Source: CAD feature listing. Evaluate the final solid. Frame: model axes, mm. A direction names the side the tool comes from. Coordinates: 2 decimals unless noted, no trailing zeros. Write each loop counter-clockwise with the first axis right and the second up, starting at its lowest first coordinate (ties: lowest second). Pieces come first, ordered by that corner, then holes. Notation, with made-up numbers: (-28.5, 10) - (-8.5, 10) arc R25 cw to (-8.5, 39) - close; hole circle Ø8 at (68.5, 86.5). An arc over 180 degrees is marked (long way). One line per question, with ' | ' between items. Start each with the question number.
Q1. Line query: line 1 (Z direction, x = 320, y = 37); line 2 (Y direction, x = 270.5, z = 3.5); line 3 (X direction, y = 23, z = 11). Output: solid intervals per line, ascending.
Q2. Draft query along Y for faces 4 (the face through (410.449, 4, 0)), 5 (the face through (251, 3, -5)). Return one class per face: +Y half, -Y half, draft (parallel to the pull), parting line (faces both ways), or undercut.
Q3. Access query for faces 1 (the face through (422, -13.242, 0)), 2 (the face through (251, 4, 5)), 3 (the face through (427.48, -8.9, 12.54)). Directions: +Z, -Z, +X, -X, +Y, -Y. A direction counts if a zero-diameter tool reaches every point of the face in a straight line with its end or side. Return the directions, or none.
Q4. Cut plane C-C, the plane z = -27. Return loops of the section in (x, y), plus the area to 3 significant figures.
Q5. Contact query for flat-ended pins moving along their axis: P1, Ø4.5, axis at x = 427, y = 5, coming from the +Z side; P2, Ø21.5, axis at x = 194.5, y = -8, coming from the -Z side; P3, Ø15.5, axis at y = 8, z = -18, coming from the -X side; P4, Ø21.5, axis at x = 174.5, y = 10, coming from the +Z side. Output: stop coordinate, or through.
Q6. Cut plane B-B, the plane x = 400.5. Return loops of the section in (y, z), plus the area to 3 significant figures.
Q7. Cut plane A-A, the plane y = 7. Return loops of the section in (x, z).
```python
from build123d import *

# Parameters (mm, degrees)
CUT_EXTRUDE1_DEPTH  = 212.88306668
BOSS_EXTRUDE2_DEPTH = 139.7
SKETCH9_R           = 35.95202499
BOSS_EXTRUDE3_DEPTH = 4
CUT_EXTRUDE2_DEPTH  = 4
SKETCH11_W          = 10
SKETCH11_H          = 34
CUT_EXTRUDE3_DEPTH  = 15


with BuildPart() as part:
    # Sketch3 → Revolve1 (revolve)
    with BuildSketch(Plane.XY):
        with BuildLine():
            Line((285.74876522, 39.710021262), (285.74876522, 3.757996272))
            Line((285.74876522, 3.757996272), (80.74876522, 3.757996272))
            Line((80.74876522, 3.757996272), (80.74876522, 19.634316044))
            add(Edge.make_bspline(
                [(80.74876522, 19.634316044), (82.347112552, 19.950400666), (85.636412123, 20.593859316), (92.311794173, 21.870421625), (109.164486257, 24.943674568), (127.867996046, 27.977765645), (146.633052135, 30.604670801), (163.733801994, 32.658467989), (174.004488004, 33.801497199), (184.284802392, 34.855212792), (194.57611333, 35.797171826), (204.876878825, 36.627240946), (213.466527777, 37.244314669), (220.34120026, 37.693162367), (227.218898943, 38.097179671), (233.238636081, 38.411453209), (238.400481516, 38.652791264), (242.701722554, 38.8352093), (246.145182192, 38.969923968), (249.584994627, 39.093417446), (253.03241088, 39.20568842), (256.467961578, 39.306735697), (259.924132141, 39.396558203), (263.346991762, 39.475154984), (266.82565511, 39.542525204), (270.211898057, 39.598668148), (273.756466178, 39.643583219), (276.60509147, 39.673059099), (279.43950326, 39.691306197), (281.597603414, 39.703938851), (283.942998009, 39.708617629), (285.03032454, 39.710021262), (285.74876522, 39.710021262)],
                knots=[0.322773044, 0.322773044, 0.322773044, 0.322773044, 0.322773044, 0.341563488, 0.3614269, 0.401153715, 0.520334158, 0.56006097, 0.579924379, 0.599787787, 0.639514601, 0.679241414, 0.699104823, 0.718968231, 0.738831638, 0.758695045, 0.778558452, 0.788490156, 0.798421859, 0.808353563, 0.818285267, 0.828216971, 0.838148675, 0.848080378, 0.858012082, 0.867943786, 0.87787549, 0.887807193, 0.897738897, 0.902704749, 0.9076706, 0.917602304, 0.917602304, 0.917602304, 0.917602304, 0.917602304], degree=4))
        make_face()
    revolve(axis=Axis((285.74876522, 3.757996272, 0), (-1, 0, 0)))

    # Sketch6 → Cut-Extrude1 (cut, through all)
    with BuildSketch(Plane(origin=(285.74876522, 0, 0), x_dir=(0, 0, -1), z_dir=(1, 0, 0))):
        with BuildLine():
            Line((-5, -31.844645496), (-5, 39.36063804))
            ThreePointArc((-5, 39.360638041), (-35.95202499, 3.757996272), (-5, -31.844645496))
        make_face()
        with BuildLine():
            ThreePointArc((35.95202499, 3.757996272), (27.132160123, 27.346001444), (5, 39.36063804))
            Line((5, 39.36063804), (5, -31.844645496))
            ThreePointArc((5, -31.844645496), (27.132160123, -19.830008899), (35.95202499, 3.757996272))
        make_face()
    extrude(amount=-CUT_EXTRUDE1_DEPTH, mode=Mode.SUBTRACT)

    # Sketch8 → Boss-Extrude2 (add)
    with BuildSketch(Plane(origin=(285.74876522, 0, 0), x_dir=(0, 0, -1), z_dir=(1, 0, 0))):
        with BuildLine():
            Line((5, -31.844645496), (5, 39.360638041))
            ThreePointArc((5, 39.360638041), (0, 39.710021262), (-5, 39.360638041))
            Line((-5, 39.360638041), (-5, -31.844645496))
            ThreePointArc((-5, -31.844645496), (0, -32.194028718), (5, -31.844645496))
        make_face()
    extrude(amount=BOSS_EXTRUDE2_DEPTH)

    # Sketch9 → Boss-Extrude3 (add)
    with BuildSketch(Plane(origin=(425.44876522, 0, 0), x_dir=(0, 0, -1), z_dir=(1, 0, 0))):
        with Locations(Location((0, 3.757996272, 0), (0, 0, 262.00572083))):
            Circle(SKETCH9_R)
    extrude(amount=BOSS_EXTRUDE3_DEPTH)

    # Sketch10 → Cut-Extrude2 (cut)
    with BuildSketch(Plane(origin=(429.44876522, 0, 0), x_dir=(0, 0, -1), z_dir=(1, 0, 0))):
        Polygon((-17, -4.442003728), (-17, 11.957996272), (-8.2, 20.757996272), (8.2, 20.757996272), (17, 11.957996272), (17, -4.442003728), (8.2, -13.242003728), (-8.2, -13.242003728), align=None)
    extrude(amount=-CUT_EXTRUDE2_DEPTH, mode=Mode.SUBTRACT)

    # Sketch11 → Cut-Extrude3 (cut)
    with BuildSketch(Plane(origin=(425.44876522, 0, 0), x_dir=(0, 0, -1), z_dir=(1, 0, 0))):
        with Locations((0, 3.757996272)):
            Rectangle(SKETCH11_W, SKETCH11_H)
    extrude(amount=-CUT_EXTRUDE3_DEPTH, mode=Mode.SUBTRACT)


solid = part.part
```
Reply:
1) line 1: z = -5 to 5 | line 2: y = -31.91 to 39.43 | line 3: x = 425.45 to 429.45
2) face 4: undercut | face 5: draft
3) face 1: +X | face 2: +Z, -X, +Y, -Y | face 3: +X, -X
4) outline: (425.45, -19.98) - (429.45, -19.98) - (429.45, 27.5) - (425.45, 27.5) - close | area: 190 mm^2
5) P1: stops at z = 35.95 | P2: stops at z = -5 | P3: stops at x = 425.45 | P4: stops at z = 5
6) outline: (-31.84, -5) - (39.36, -5) arc R35.95 ccw to (39.36, 5) - (-31.84, 5) arc R35.95 ccw to start | area: 717 mm^2
7) outline: (80.75, -5) - (410.45, -5) - (410.45, 5) - (80.75, 5) - close; (425.45, -35.81) - (429.45, -35.81) - (429.45, -17) - (425.45, -17) - close; (425.45, 17) - (429.45, 17) - (429.45, 35.81) - (425.45, 35.81) - close
